Read the model definition and answer for the solid it produces. Units are mm, in the model's axes. A direction names the side the tool comes from. Give positions to 0.01 mm unless a question says otherwise; leave off trailing zeros. Loops run counter-clockwise (first coordinate to the right, second up) from the corner with the lowest first, then second, coordinate; pieces in that order, holes last. Notation, with made-up numbers: (-30.75, -20.75) - (-11.75, -20.75) arc R15 cw to (-11.75, 8.25) - close; hole circle Ø3 at (34.25, 18.25). An arc over 180 degrees is marked (long way). Use a Markdown table: item, result. Add a question column.
Item 1: A cutting plane is placed at A-A (y = 4). Determine the outline of the cut face in (x, z).
Item 2: For a pull along X with two mould halves and no side action, classify faces 5 (the face through (12, 0, 2)), 6 (the face through (0, 19.6, 4)), 7 (the face through (17.5, -3, 1)) as +X half, -X half, draft (parallel to the pull), parting line (faces both ways), or undercut.
Item 3: A cutting plane is placed at B-B (z = 1.25). Determine the outline of the cut face in (x, y).
Item 4: A cutting plane is placed at D-D (z = 4.6). Determine the outline of the cut face in (x, y), plus the area to 3 significant figures.
Item 5: Which of the six approach directions +Z, -Z, +X, -X, +Y, -Y give full straight-line access (tool end or side, diameter ignored) to faces 1 (the face through (10, -30, 1)), 2 (the face through (11, 0, 1)), 3 (the face through (0, -18, 4)), 4 (the face through (-15.1, 0, 4))?
Item 6: A cutting plane is placed at C-C (x = -10). Determine the outline of the cut face in (y, z).
Item 7: Each of these flat-tipped pins is pushed along its axis until it touches: P1, Ø4, axis at x = 0, y = -30, coming from the +Z side; P2, Ø2, axis at x = -7, z = 1.5, coming from the +Y side; P3, Ø1.5, axis at y = -7, z = 5, coming from the -X side. Where does it stop, or does it pass through?
Item 8: Consider probe 1 along Y at (x, z) = (0, 1.3); probe 2 along Y at (x, z) = (11, 3.4); probe 3 along X at (y, z) = (8, 0.35). Determine where each line is inside the solid, lowest interval first. Write a range as [from, to].
from build123d import *

# Parameters (mm, degrees)
SKETCH_R      = 1.75
SKETCH_W      = 22
SKETCH_H      = 30
PAD_DEPTH     = 2
SKETCH001_W   = 30.2
SKETCH001_H   = 39.2
SKETCH001_W_2 = 27
SKETCH001_H_2 = 36
PAD001_DEPTH  = 6


with BuildPart() as part:
    # Sketch → Pad (new body)
    with BuildSketch(Plane.XY):
        with BuildLine():
            ThreePointArc((3.5, 25), (0, 28.5), (-3.5, 25))
            Line((-3.5, 25), (-17.5, 25))
            Line((-17.5, 25), (-17.5, -30))
            Line((-17.5, -30), (-3.5, -30))
            ThreePointArc((-3.5, -30), (0, -33.5), (3.5, -30))
            Line((3.5, -30), (17.5, -30))
            Line((17.5, -30), (17.5, 25))
            Line((17.5, 25), (3.5, 25))
        make_face()
        with Locations((0, 25)):
            Circle(SKETCH_R, mode=Mode.SUBTRACT)
        with Locations((0, -30)):
            Circle(SKETCH_R, mode=Mode.SUBTRACT)
        Rectangle(SKETCH_W, SKETCH_H, mode=Mode.SUBTRACT)
    extrude(amount=PAD_DEPTH)

    # Sketch001 → Pad001 (join)
    with BuildSketch(Plane.XY):
        Rectangle(SKETCH001_W, SKETCH001_H)
        Rectangle(SKETCH001_W_2, SKETCH001_H_2, mode=Mode.SUBTRACT)
    extrude(amount=PAD001_DEPTH)


solid = part.part
Geometry says:
| question | item | result |
|---|---|---|
| 1 | outline | (-17.5, 0) - (-11, 0) - (-11, 2) - (-13.5, 2) - (-13.5, 6) - (-15.1, 6) - (-15.1, 2) - (-17.5, 2) - close; (11, 0) - (17.5, 0) - (17.5, 2) - (15.1, 2) - (15.1, 6) - (13.5, 6) - (13.5, 2) - (11, 2) - close |
| 2 | face 5 | undercut |
| 2 | face 6 | draft |
| 2 | face 7 | +X half |
| 3 | outline | (-17.5, -30) - (-3.5, -30) arc R3.5 ccw to (3.5, -30) - (17.5, -30) - (17.5, 25) - (3.5, 25) arc R3.5 ccw to (-3.5, 25) - (-17.5, 25) - close; hole (-11, -15) - (11, -15) - (11, 15) - (-11, 15) - close; hole circle Ø3.5 at (0, -30); hole circle Ø3.5 at (0, 25) |
| 4 | outline | (-15.1, -19.6) - (15.1, -19.6) - (15.1, 19.6) - (-15.1, 19.6) - close; hole (-13.5, -18) - (13.5, -18) - (13.5, 18) - (-13.5, 18) - close |
| 4 | area | 212 mm² |
| 5 | face 1 | +Z, -Z, +X, -Y |
| 5 | face 2 | +Z, -Z |
| 5 | face 3 | +Z |
| 5 | face 4 | +Z, -X, +Y, -Y |
| 6 | outline | (-30, 0) - (-15, 0) - (-15, 2) - (-18, 2) - (-18, 6) - (-19.6, 6) - (-19.6, 2) - (-30, 2) - close; (15, 0) - (25, 0) - (25, 2) - (19.6, 2) - (19.6, 6) - (18, 6) - (18, 2) - (15, 2) - close |
| 7 | P1 | z = 2 |
| 7 | P2 | y = 25 |
| 7 | P3 | x = -15.1 |
| 8 | probe 1 | [-33.5, -31.75], [-28.25, -15], [15, 23.25], [26.75, 28.5] |
| 8 | probe 2 | [-19.6, -18], [18, 19.6] |
| 8 | probe 3 | [-17.5, -11], [11, 17.5] |
